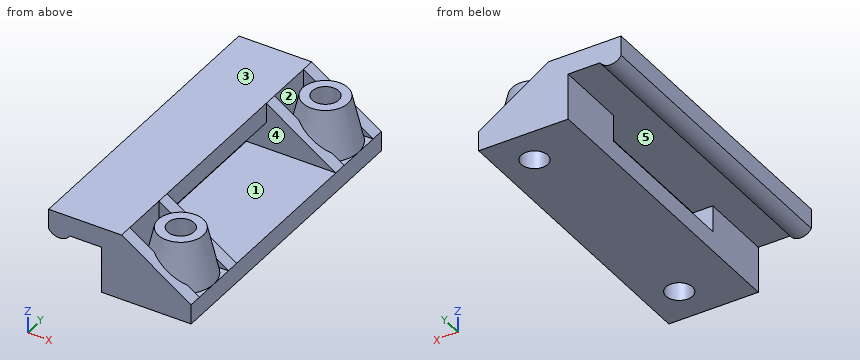
from build123d import *

# Parameters (mm, degrees)
F0_W      = 3
F0_H      = 4
F1_DEPTH  = 11
F2_DEPTH  = 2
F4_DEPTH  = 2
F5_R      = 2
F6_DEPTH  = 25
F7_R      = 3.4
F7_R_2    = 2
F8_DEPTH  = 7
F13_DEPTH = 24


with BuildPart() as f1:
    # F0 (on Front) → F1 (new body)
    with BuildSketch(Plane.XZ):
        Polygon((12, -5), (12, -2), (1.5, -2), (-1.5, -2), (-1.5, -4), (-1.5, -5), (1.5, -5), align=None)
        with BuildLine():
            Line((1.5, 4), (1.5, 5))
            Line((1.5, 5), (-9.5, 5))
            Line((-9.5, 5), (-9.5, 2))
            ThreePointArc((-9.5, 2), (-7.9057595357, 1.1241546177), (-6.3115190715, 2))
            Line((-6.3115190715, 2), (-1.5, 2))
            Line((-1.5, 2), (1.5, 2))
            Line((1.5, 2), (1.5, 4))
        make_face()
        Rectangle(F0_W, F0_H)
    extrude(amount=F1_DEPTH)

    # F0 (on Front) → F2 (join)
    with BuildSketch(Plane.XZ):
        Polygon((12, -2), (1.5, 5), (1.5, 4), (1.5, 2), (1.5, -2), align=None)
    extrude(amount=F2_DEPTH)

    # F3 (on face) → F4 (join)
    with BuildSketch(Plane.XZ.offset(11)):
        Polygon((1.5, -2), (12, -2), (1.5, 5), align=None)
    extrude(amount=-F4_DEPTH)

    # F5 (on face) → F6 (cut)
    with BuildSketch(Plane(origin=(0, 0, -5), x_dir=(1, 0, 0), z_dir=(0, 0, -1))):
        with Locations((7.0000002161, 5.5)):
            Circle(F5_R)
    extrude(amount=-F6_DEPTH, mode=Mode.SUBTRACT)

    # F7 (on face) → F8 (join)
    with BuildSketch(Plane.XY.offset(-2)):
        with Locations((7.0000002161, -5.5)):
            Circle(F7_R)
        with Locations((7.0000002161, -5.5)):
            Circle(F7_R_2, mode=Mode.SUBTRACT)
    extrude(amount=F8_DEPTH)

    # F10 (on offset) → F11 (revolve)
    with BuildSketch(Plane.YZ.offset(7)):
        Polygon((-2.1, 5), (-2.1, -2), (-2, -2), (-0.5000002161, -2), align=None)
    revolve(axis=Axis((7, -5.5, 1.7165149804), (0, 0, 1)))


with BuildPart() as f12_1:
    # F12: copy of F1
    add(f1.part.moved(Location((0, 35, 0))))


with BuildPart() as f1_1:
    add(f1.part)

    add(f12_1.part)  # F13 merges F12_1
    # F0 (on Front) → F13 (join)
    with BuildSketch(Plane.XZ):
        Polygon((12, -5), (12, -2), (1.5, -2), (-1.5, -2), (-1.5, -4), (-1.5, -5), (1.5, -5), align=None)
        with BuildLine():
            Line((1.5, 4), (1.5, 5))
            Line((1.5, 5), (-9.5, 5))
            Line((-9.5, 5), (-9.5, 2))
            ThreePointArc((-9.5, 2), (-7.9057595357, 1.1241546177), (-6.3115190715, 2))
            Line((-6.3115190715, 2), (-1.5, 2))
            Line((-1.5, 2), (1.5, 2))
            Line((1.5, 2), (1.5, 4))
        make_face()
    extrude(amount=-F13_DEPTH)


solid = f1_1.part
For this review, take the finished solid that the model builds, in its own axes (mm). Face numbers are marked on the shaded views. A direction names the side the tool comes from. Coordinates: 2 decimals unless noted, no trailing zeros. Loops run counter-clockwise (first coordinate to the right, second up) from the corner with the lowest first, then second, coordinate; pieces in that order, holes last. Notation, with made-up numbers: (76, -12) - (131, -12) arc R23 cw to (131, 22) - close; hole circle Ø1 at (37, 76.5). An arc over 180 degrees is marked (long way). Return JSON: item names as keys, results as strings.
Item 1: Take a section at A-A (y = 21). Give the boundary of the cut face in (x, z), then the cut area to 3 significant figures.
Determined:
{"outline": "(-9.5, 2) arc R1.89 ccw to (-6.31, 2) - (1.5, 2) - (1.5, 5) - (-9.5, 5) - close; (-1.5, -5) - (12, -5) - (12, -2) - (-1.5, -2) - close", "area": "75.5 mm2"}
Item 2: Insertion check: pin 1 (4 mm diameter, centred on x = 4.5, y = 8, fed in from +Z); pin 2 (4 mm diameter, centred on y = 15.5, z = 2, fed in from +X); pin 3 (1 mm diameter, centred on y = 8.5, z = -0.5, fed in from -X); pin 4 (2 mm diameter, centred on y = 19.5, z = -2, fed in from -X). Each pin has a flat end and moves straight along its axis. Give the tip position at first contact, or say it passes through.
Determined:
{"pin 1": "stops at z = -2", "pin 2": "stops at x = 1.5", "pin 3": "passes through", "pin 4": "stops at x = -1.5"}
Item 3: For line 1 (Y direction, x = 3, z = 3.5); line 2 (Y direction, x = 7, z = 0.25); line 3 (Y direction, x = 7, z = -3.25), list the stretches that pass through material, from the lowest coordinate up.
Determined:
{"line 1": "y = -11 to -9, -2 to 0, 24 to 26, 33 to 35", "line 2": "y = -11 to -7.5, -3.5 to 0, 24 to 27.5, 31.5 to 35", "line 3": "y = -11 to -7.5, -3.5 to 27.5, 31.5 to 35"}
Item 4: Mouldability with a two-part tool opening along X and no side actions: class the marked faces 4 and 5 as pulls with the +X half, pulls with the -X half, needs draft (parallel to the pull), parting line crosses it, or undercut.
Determined:
{"face 4": "needs draft", "face 5": "undercut"}
Item 5: Take a section at D-D (x = 7). Give the boundary of the cut face in (y, z).
Determined:
{"outline": "(-11, -5) - (-7.5, -5) - (-7.5, 5) - (-8.9, 5) - (-9.74, 1.33) - (-11, 1.33) - close; (-3.5, -5) - (27.5, -5) - (27.5, 5) - (26.1, 5) - (25.26, 1.33) - (24, 1.33) - (24, -2) - (0, -2) - (0, 1.33) - (-1.26, 1.33) - (-2.1, 5) - (-3.5, 5) - close; (31.5, -5) - (35, -5) - (35, 1.33) - (33.74, 1.33) - (32.9, 5) - (31.5, 5) - close"}
Item 6: Take a section at B-B (x = 0). Give the boundary of the cut face in (y, z).
Determined:
{"outline": "(-11, -5) - (35, -5) - (35, 5) - (-11, 5) - close; hole (0, -2) - (24, -2) - (24, 2) - (0, 2) - close"}
Item 7: For the marked faces 1, 2 and 3, list the 3-axis set-ups (+Z, -Z, +X, -X, +Y, -Y) from which the entire face can be reached by the end or side of a thin tool; tool diameter is ignored.
Determined:
{"face 1": "+X, -X", "face 2": "+Z", "face 3": "+Z, +X, -X, +Y, -Y"}
Item 8: Take a section at C-C (z = 3). Give the boundary of the cut face in (x, y), then the cut area to 3 significant figures.
Determined:
{"outline": "(-9.5, -11) - (4.5, -11) - (4.5, -9) - (1.5, -9) - (1.5, -2) - (4.5, -2) - (4.5, 0) - (1.5, 0) - (1.5, 24) - (4.5, 24) - (4.5, 26) - (1.5, 26) - (1.5, 33) - (4.5, 33) - (4.5, 35) - (-9.5, 35) - close; circle Ø7.71 at (7, -5.5); circle Ø7.71 at (7, 29.5); hole circle Ø4 at (7, -5.5); hole circle Ø4 at (7, 29.5)", "area": "598 mm2"}
